Answer from the drawing. Dimensions are ordinates in mm from the lowest x, y and z of the part. Coordinates: 2 decimals unless noted, no trailing zeros. Write each loop counter-clockwise with the first axis right and the second up, starting at its lowest first coordinate (ties: lowest second). Pieces come first, ordered by that corner, then holes.
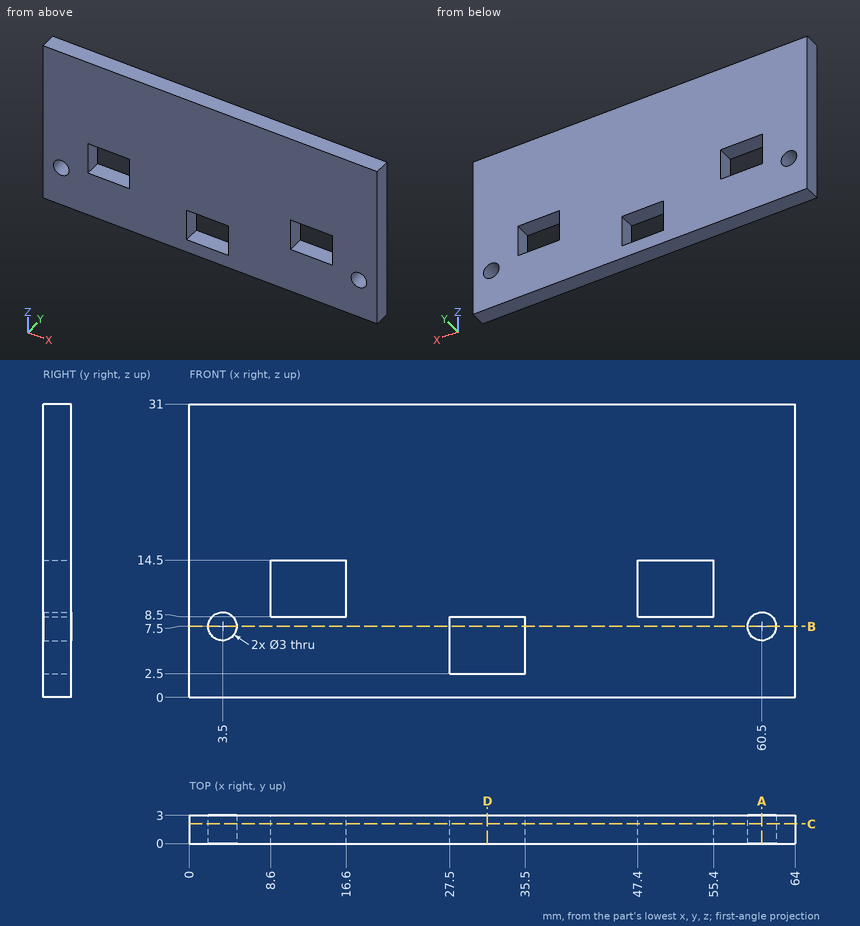
(1) Section C-C, the plane y = 2.1 is taken. Write down the section's boundary in (x, z).
(2) Section A-A, the plane x = 60.5 is taken. Write down the section's boundary in (y, z).
(3) Section B-B, the plane z = 7.5 is taken. Write down the section's boundary in (x, y), plus the area to 3 significant figures.
(4) Find the intervals of material crossed by probe 1 along X at (y, z) = (2.05, 7.5); probe 2 along X at (y, z) = (0.6, 3.5); probe 3 along Z at (x, y) = (29, 2.2), in increasing order.
(5) Section D-D, the plane x = 31.5 is taken. Write down the section's boundary in (y, z), plus the area to 3 significant figures.
Solution:
1. outline: (0, 0) - (64, 0) - (64, 31) - (0, 31) - close; hole circle Ø3 at (3.5, 7.5); hole (8.6, 8.5) - (16.6, 8.5) - (16.6, 14.5) - (8.6, 14.5) - close; hole (27.5, 2.5) - (35.5, 2.5) - (35.5, 8.5) - (27.5, 8.5) - close; hole (47.4, 8.5) - (55.4, 8.5) - (55.4, 14.5) - (47.4, 14.5) - close; hole circle Ø3 at (60.5, 7.5)
2. outline: (0, 0) - (3, 0) - (3, 6) - (0, 6) - close; (0, 9) - (3, 9) - (3, 31) - (0, 31) - close
3. outline: (0, 0) - (2, 0) - (2, 3) - (0, 3) - close; (5, 0) - (27.5, 0) - (27.5, 3) - (5, 3) - close; (35.5, 0) - (59, 0) - (59, 3) - (35.5, 3) - close; (62, 0) - (64, 0) - (64, 3) - (62, 3) - close
3. area: 150 mm2
4. probe 1: x = 0 to 2, 5 to 27.5, 35.5 to 59, 62 to 64
4. probe 2: x = 0 to 27.5, 35.5 to 64
4. probe 3: z = 0 to 2.5, 8.5 to 31
5. outline: (0, 0) - (3, 0) - (3, 2.5) - (0, 2.5) - close; (0, 8.5) - (3, 8.5) - (3, 31) - (0, 31) - close
5. area: 75.0 mm2
